Verification items for the finished model (mm, model axes). Face numbers are marked on the shaded views. A direction names the side the tool comes from. Round coordinates to 2 decimals unless told otherwise and drop trailing zeros. Order: outer loops, then holes, each group sorted by start corner. A loop starts at its lowest first (then second) coordinate and runs counter-clockwise, first axis right, second up. Notation, with made-up numbers: M 73,-12.75 L 94,-12.75 A17 cw 94,-1.75 Z; hole C 63,-20.5 d7. An arc over 180 degrees is marked long. Use one line per item in the form item = value. Start each with the question number.
Item 1: Cross-section at C-C on y = 4.5. Enter the section's corners in (x, z), then the cut area to 3 significant figures.
Item 2: Cross-section at D-D on y = 26. Enter the section's corners in (x, z), then the cut area to 3 significant figures.
Item 3: Go/stop test with flat-tipped pins: pin 1 Ø3.5 at (x, z) = (17.68, -17.68) entering from -Y; pin 2 Ø1 at (x, z) = (-18, -4) entering from -Y; pin 3 Ø4 at (x, y) = (-3.5, 14.5) entering from +Z; pin 4 Ø6 at (y, z) = (13.5, 15) entering from -X. Record where each tip stops, or that it passes through.
Item 4: Thickness scan on probe 1 along Y at (x, z) = (-12, -13); probe 2 along Z at (x, y) = (-3.5, -0.5); probe 3 along X at (y, z) = (23.5, 11.5). Record the ranges inside material, lowest first. Write a range as [from, to].
Item 5: Cross-section at A-A on z = 0. Enter the section's corners in (x, y), then the cut area to 3 significant figures.
Item 6: Tool access check on the marked faces 1, 2 and 3. Record the directions out of +Z, -Z, +X, -X, +Y, -Y that give a thin tool (end or side, any length) a straight path to the whole face; none if there is none.
Item 7: Cross-section at B-B on x = 0. Enter the section's corners in (y, z).
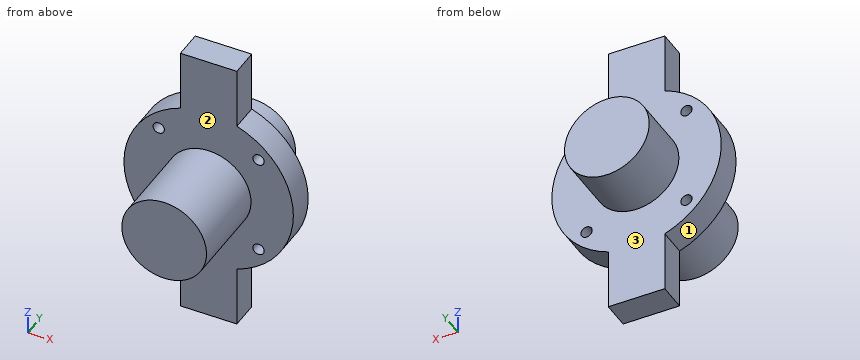
from build123d import *
from build123d.topology import SkipClean

# Parameters (mm, degrees)
SKETCH1_R           = 30
SKETCH1_R_2         = 15
SKETCH1_R_3         = 2
BOSS_EXTRUDE1_DEPTH = 10
BOSS_EXTRUDE2_START = -10
BOSS_EXTRUDE2_DEPTH = 10
SKETCH5_R           = 15
BOSS_EXTRUDE3_DEPTH = 30


with BuildPart() as part:
    # Sketch1 → Boss-Extrude1 (new body)
    with BuildSketch(Plane(origin=(0, 0, 0), x_dir=(1, 0, 0), z_dir=(0, 1, 0))):
        with Locations(Location((0, 0, 0), (0, 0, 270))):
            Circle(SKETCH1_R)
        with Locations(Location((0, 0, 0), (0, 0, 270))):
            Circle(SKETCH1_R_2, mode=Mode.SUBTRACT)
        with Locations(Location((-17.67766953, 17.67766953, 0), (0, 0, 270))):
            Circle(SKETCH1_R_3, mode=Mode.SUBTRACT)
        with Locations(Location((17.67766953, 17.67766953, 0), (0, 0, 270))):
            Circle(SKETCH1_R_3, mode=Mode.SUBTRACT)
        with Locations(Location((17.67766953, -17.67766953, 0), (0, 0, 270))):
            Circle(SKETCH1_R_3, mode=Mode.SUBTRACT)
        with Locations(Location((-17.67766953, -17.67766953, 0), (0, 0, 270))):
            Circle(SKETCH1_R_3, mode=Mode.SUBTRACT)
    extrude(amount=BOSS_EXTRUDE1_DEPTH)

    # Sketch2 → Boss-Extrude2 (add)
    with SkipClean():  # the faces are left unmerged after this step: merging them gives an invalid solid
        with BuildSketch(Plane(origin=(0, 10, 0), x_dir=(1, 0, 0), z_dir=(0, 1, 0)).offset(BOSS_EXTRUDE2_START)):
            with BuildLine():
                ThreePointArc((-10, 11.180339887), (0, 15), (10, 11.180339887))
                Line((10, 11.180339887), (10, 28.284271247))
                ThreePointArc((10, 28.284271247), (0, 30), (-10, 28.284271247))
                Line((-10, 28.284271247), (-10, 11.180339887))
            make_face()
            with BuildLine():
                ThreePointArc((-10, 28.284271247), (0, 30), (10, 28.284271247))
                Line((10, 28.284271247), (10, 50))
                Line((10, 50), (-10, 50))
                Line((-10, 50), (-10, 28.284271247))
            make_face()
            with BuildLine():
                ThreePointArc((10, -11.180339887), (0, -15), (-10, -11.180339887))
                Line((-10, -11.180339887), (-10, -28.284271247))
                ThreePointArc((-10, -28.284271247), (0, -30), (10, -28.284271247))
                Line((10, -28.284271247), (10, -11.180339887))
            make_face()
            with BuildLine():
                Line((10, -50), (10, -28.284271247))
                ThreePointArc((10, -28.284271247), (0, -30), (-10, -28.284271247))
                Line((-10, -28.284271247), (-10, -50))
                Line((-10, -50), (10, -50))
            make_face()
        extrude(amount=BOSS_EXTRUDE2_DEPTH)

    # Sketch5 → Boss-Extrude3 (add, symmetric)
    with BuildSketch(Plane(origin=(0, 0, 0), x_dir=(1, 0, 0), z_dir=(0, 1, 0))):
        with Locations(Location((0, 0, 0), (0, 0, 270))):
            Circle(SKETCH5_R)
    extrude(amount=BOSS_EXTRUDE3_DEPTH, both=True)


solid = part.part
Output values:
q1.outline = M -10,-50 L 10,-50 L 10,-28.28 A30 ccw 10,28.28 L 10,50 L -10,50 L -10,28.28 A30 ccw -10,-28.28 Z; hole C -17.68,-17.68 d4; hole C -17.68,17.68 d4; hole C 17.68,-17.68 d4; hole C 17.68,17.68 d4
q1.area = 3,600 mm2
q2.outline = C 0,0 d30
q2.area = 707 mm2
q3.pin_1 = through
q3.pin_2 = 0
q3.pin_3 = 14.92
q3.pin_4 = -9
q4.probe_1 = [0, 10]
q4.probe_2 = [-14.59, 14.59]
q4.probe_3 = [-9.63, 9.63]
q5.outline = M -30,0 L -15,0 L -15,-30 L 15,-30 L 15,0 L 30,0 L 30,10 L 15,10 L 15,30 L -15,30 L -15,10 L -30,10 Z
q5.area = 2,100 mm2
q6.face_1 = -X, +Y, -Y
q6.face_2 = -Y
q6.face_3 = +Y
q7.outline = M -30,-15 L 0,-15 L 0,-50 L 10,-50 L 10,-15 L 30,-15 L 30,15 L 10,15 L 10,50 L 0,50 L 0,15 L -30,15 Z
